Input: dimensioned drawing with shaded views. Units: mm. Origin: part minimum x, y, z. A direction names the side the tool comes from. Round coordinates to 2 decimals unless told otherwise and drop trailing zeros. Write each loop counter-clockwise with the first axis right and the second up, starting at its lowest first coordinate (ties: lowest second). Pieces come first, ordered by that corner, then holes. Notation, with made-up numbers: (54, 20) -> (63, 20) arc R16 cw to (63, 29) -> close; hole circle Ø6 at (12, -21.5). An arc over 180 degrees is marked (long way). One line per item, written item: value. Start each with the question number.
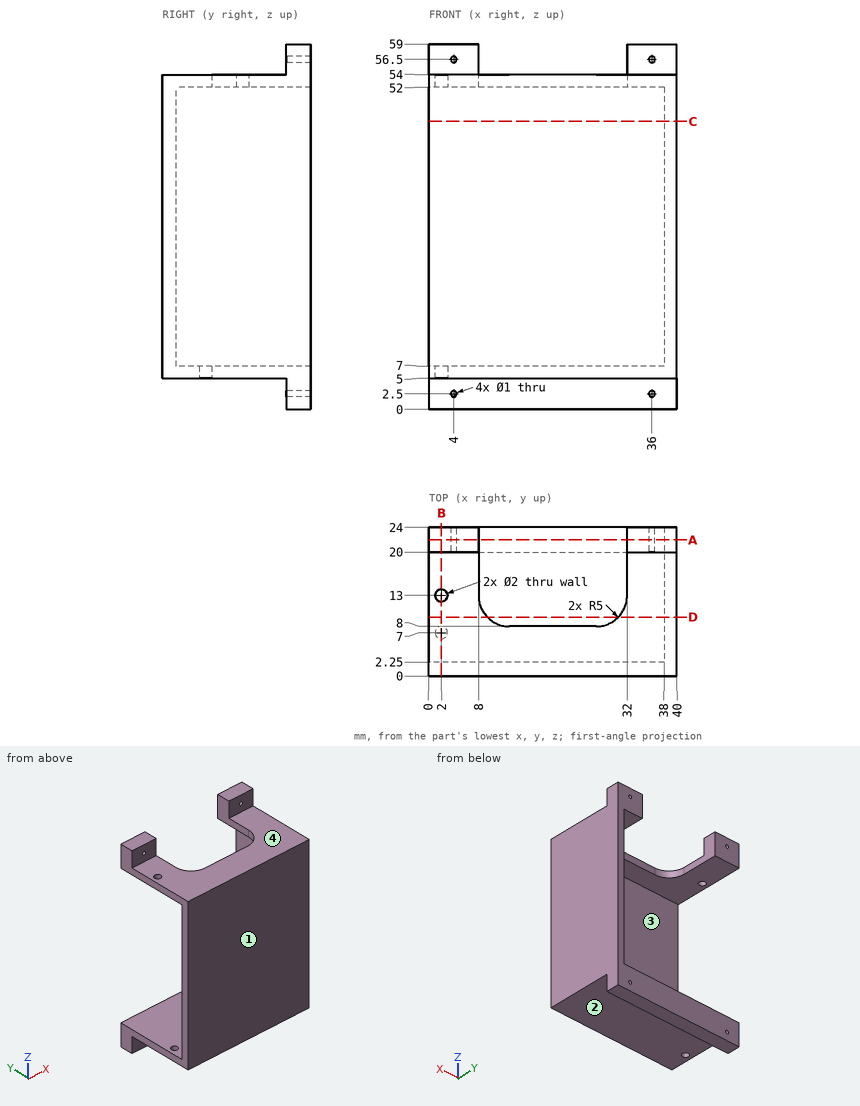
(1) Section query C-C (z = 46.5). Output: boundary loops of the cut face in (x, y), and give its area (4 significant figures).
(2) Set-up query: the marked faces 1, 2, 3 and 4. Return all of +Z, -Z, +X, -X, +Y, -Y with unobstructed straight access to the full face (end or side cutting, diameter ignored); none if empty.
(3) Pin query (flat end, axial travel): pin 1 (4 mm diameter, centred on x = 9, z = 44, fed in from +Y); pin 2 (6.5 mm diameter, centred on x = 19.5, y = 17.5, fed in from +Z); pin 3 (2.5 mm diameter, centred on x = 38, z = 56.5, fed in from -Y). Return the tip coordinate at first contact, or that it passes through.
(4) Line query: probe 1 along Z at (x, y) = (36, 21.3); probe 2 along X at (y, z) = (23.1, 56.5); probe 3 along X at (y, z) = (13, 52.45). Output: solid intervals per line, ascending.
(5) Section query A-A (y = 22). Output: boundary loops of the cut face in (x, z).
(6) Section query D-D (y = 9.5). Output: boundary loops of the cut face in (x, z).
(7) Section query B-B (x = 2). Output: boundary loops of the cut face in (y, z), and give its area (3 significant figures).
Results list:
1. outline: (0, 0) -> (40, 0) -> (40, 24) -> (38, 24) -> (38, 2.25) -> (0, 2.25) -> close
1. area: 133.5 mm^2
2. face 1: +Z, -Z, +X, -X, -Y
2. face 2: -Z, +X, -X, -Y
2. face 3: -X, +Y
2. face 4: +Z, +X, -X, -Y
3. pin 1: stops at y = 2.25
3. pin 2: stops at z = 7
3. pin 3: stops at y = 20
4. probe 1: z = 0 to 2, 3 to 7, 52 to 56, 57 to 59
4. probe 2: x = 0 to 3.5, 4.5 to 8, 32 to 35.5, 36.5 to 40
4. probe 3: x = 0 to 1, 3 to 8, 32 to 40
5. outline: (0, 0) -> (40, 0) -> (40, 59) -> (32, 59) -> (32, 52) -> (38, 52) -> (38, 7) -> (0, 7) -> close; (0, 52) -> (8, 52) -> (8, 59) -> (0, 59) -> close; hole circle Ø1 at (4, 2.5); hole circle Ø1 at (4, 56.5); hole circle Ø1 at (36, 2.5); hole circle Ø1 at (36, 56.5)
6. outline: (0, 5) -> (40, 5) -> (40, 54) -> (30.57, 54) -> (30.57, 52) -> (38, 52) -> (38, 7) -> (0, 7) -> close; (0, 52) -> (9.43, 52) -> (9.43, 54) -> (0, 54) -> close
7. outline: (0, 5) -> (6, 5) -> (6, 7) -> (2.25, 7) -> (2.25, 52) -> (12, 52) -> (12, 54) -> (0, 54) -> close; (8, 5) -> (20, 5) -> (20, 0) -> (24, 0) -> (24, 7) -> (8, 7) -> close; (14, 52) -> (24, 52) -> (24, 59) -> (20, 59) -> (20, 54) -> (14, 54) -> close
7. area: 229 mm^2
